from build123d import *

# Parameters (mm, degrees)
F2_DEPTH = 5
F3_SIZE  = 2


with BuildPart() as f1:
    # F0 (on Front) → F1 (revolve)
    with BuildSketch(Plane.XZ):
        Polygon((-6.9665953279, 11.8032604518), (-4.6637503628, 7.9016302259), (-1.741648832, 7.9016302259), (0, 7.9016302259), (0, 20.5576719715), (-5.0148367882, 20.5576719715), (-17.2530292513, 18.8067907016), (-12.438103174, 13.5541430143), align=None)
        Polygon((-5.0148367882, 20.5576719715), (0, 20.5576719715), (0, 25.5600530654), (-2.0939521492, 25.5600530654), (-2.5074183941, 22.3113913089), align=None)
        Polygon((-1.741648832, 7.9016302259), (-4.6637503628, 7.9016302259), (-2.3318751814, 6.6709434614), (-2.3318751814, 5.9016302259), (0, 5.9016302259), (0, 7.9016302259), align=None)
        Polygon((-2.3318751814, 5.9016302259), (0, 1.9508151129), (0, 5.9016302259), align=None)
    revolve(axis=Axis((0, 0, 10.2788359857), (0, 0, -1)))

    # F2 (add): a face of the model
    f2_faces = [f1.faces().sort_by_distance(p)[0] for p in [
        (0, 0, 25.5600530654),
    ]]
    extrude(f2_faces, amount=F2_DEPTH)

    # F3
    f3_edges = [f1.edges().sort_by_distance(p)[0] for p in [
        (2.093952, 0, 30.560053),
    ]]
    chamfer(f3_edges, length=F3_SIZE)


solid = f1.part
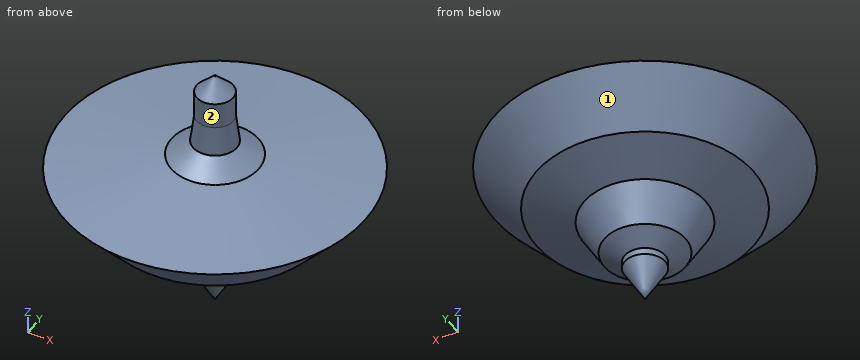
The model under review builds one solid part; all positions refer to its coordinate system, in mm. Face numbers are marked on the shaded views. A direction names the side the tool comes from. Give positions to 0.01 mm unless a question says otherwise; leave off trailing zeros. Write each loop counter-clockwise with the first axis right and the second up, starting at its lowest first coordinate (ties: lowest second). Pieces come first, ordered by that corner, then holes.
1. For P1, Ø3, axis at x = -9.5, y = 5.5, coming from the +Z side; P2, Ø6, axis at x = 6, y = -9.5, coming from the -Z side; P3, Ø10, axis at x = 0, y = 6.5, coming from the -Z side; P4, Ø12, axis at x = 1.5, y = 0.5, coming from the -Z side, all flat-tipped, find the tip position at first contact; note any pin that passes through.
2. Wall thickness on L1, parallel to X at y = -4, z = 15; L2, parallel to Y at x = -12.5, z = 18; L3, parallel to X at y = 1.5, z = 15.25: over which ranges is each line inside the solid? List them lowest first.
3. Add section A-A, the plane z = 4.25. Write out the cut boundary in (x, y).
4. Tool access review of the marked faces 1 and 2: name each direction out of +Z, -Z, +X, -X, +Y, -Y from which nothing blocks a thin tool from reaching the whole face with its end or side.
5. Add section B-B, the plane z = 10.5. Write out the cut boundary in (x, y), plus the area to 3 significant figures.
Worked answers:
1. P1: stops at z = 19.92
1. P2: stops at z = 12.21
1. P3: stops at z = 4.49
1. P4: stops at z = 1.95
2. L1: x = -13.17 to 13.17
2. L2: y = -10.79 to 10.79
2. L3: x = -13.91 to 13.91
3. outline: circle Ø2.71 at (0, 0)
4. face 1: -Z
4. face 2: +Z
5. outline: circle Ø12.39 at (0, 0)
5. area: 121 mm2
